Geometry check sheet. Reference: the model listing, model coordinates, mm. Round coordinates to 2 decimals unless told otherwise and drop trailing zeros. Order: outer loops, then holes, each group sorted by start corner. A loop starts at its lowest first (then second) coordinate and runs counter-clockwise, first axis right, second up.
(1) Sectioned sample at C-C (x = -2). Record the boundary of the cut face in (y, z).
(2) Go/stop test with flat-tipped pins: pin 1 (1.5 mm diameter, centred on y = -18.5, z = 42, fed in from -X); pin 2 (6 mm diameter, centred on y = -1, z = 70, fed in from -X); pin 3 (8 mm diameter, centred on x = -19.5, z = 38, fed in from -Y); pin 4 (10 mm diameter, centred on x = 3.5, z = 85, fed in from +Y). Record where each tip stops, or that it passes through.
(3) Material ranges on line 1 along Y through (x, z) = (0, 60); line 2 along Z through (x, y) = (-5, -5); line 3 along Y through (x, z) = (22, 77.5), recorded low to high.
(4) Sectioned sample at A-A (y = 13). Record the boundary of the cut face in (x, z).
(5) Release check for a two-part mould opening along Y. For faces 1 (the face through (22.015, -1.678, 83.496)), 2 (the face through (-22.05, -1.73, 39.43)), 3 (the face through (0.35, -5.206, 54.627)) record: +Y half, -Y half, draft (parallel to the pull), parting line (faces both ways), or undercut.
(6) Sectioned sample at B-B (x = 11). Record the boundary of the cut face in (y, z).
from build123d import *

# Parameters (mm, degrees)
F0_R          = 25
F1_DEPTH      = 140
F1_DEPTH_BACK = 140
F3_DEPTH      = 70
F3_DEPTH_BACK = 70
F4_R          = 4
F5_DEPTH      = 100


with BuildPart() as f1:
    # F0 (on Top) → F1 (new body, two sides)
    with BuildSketch(Plane.XY) as f1_sk:
        Circle(F0_R)
        Polygon((-17.759334, -15.390129), (-17.467051, -11.30056), (-13.377482, -11.592843), (-13.669765, -15.682412), align=None, mode=Mode.SUBTRACT)
        Polygon((-4.986074, -16.984997), (-3.020925, -20.583356), (-6.619284, -22.548505), (-8.584433, -18.950146), align=None, mode=Mode.SUBTRACT)
        Polygon((-12.70393, -19.770184), (-13.575676, -15.763931), (-9.569424, -14.892185), (-8.697678, -18.898437), align=None, mode=Mode.SUBTRACT)
        Polygon((-16.101728, -7.354277), (-17.534361, -11.195835), (-21.375918, -9.763202), (-19.943286, -5.921645), align=None, mode=Mode.SUBTRACT)
        Polygon((-17.52145, -2.519885), (-19.978364, -5.802198), (-23.260677, -3.345284), (-20.803763, -0.062972), align=None, mode=Mode.SUBTRACT)
        Polygon((2.900576, -20.60066), (0.001641, -23.5), (-2.8977, -20.601065), (0.001236, -17.701724), align=None, mode=Mode.SUBTRACT)
        Polygon((8.587079, -18.948947), (6.622432, -22.547581), (3.023799, -20.582934), (4.988446, -16.9843), align=None, mode=Mode.SUBTRACT)
        Polygon((12.70669, -19.76841), (8.700316, -18.897223), (9.571503, -14.890849), (13.577877, -15.762036), align=None, mode=Mode.SUBTRACT)
        Polygon((13.379101, -11.590975), (17.468628, -11.298121), (17.761482, -15.387649), (13.671955, -15.680503), align=None, mode=Mode.SUBTRACT)
        Polygon((21.377281, -9.760218), (17.535924, -11.193387), (16.102755, -7.352029), (19.944112, -5.91886), align=None, mode=Mode.SUBTRACT)
        Polygon((19.979174, -5.799408), (17.521802, -2.517439), (20.803772, -0.060067), (23.261143, -3.342037), align=None, mode=Mode.SUBTRACT)
        Polygon((-23.26091, 3.343661), (-19.978769, 5.800803), (-17.521626, 2.518662), (-20.803767, 0.061519), align=None, mode=Mode.SUBTRACT)
        Polygon((-19.943699, 5.920253), (-21.3766, 9.76171), (-17.535142, 11.194611), (-16.102242, 7.353153), align=None, mode=Mode.SUBTRACT)
        Polygon((-13.67086, 15.681458), (-13.378291, 11.59191), (-17.467839, 11.299341), (-17.760408, 15.388889), align=None, mode=Mode.SUBTRACT)
        Polygon((-9.570464, 14.891517), (-13.576777, 15.762984), (-12.70531, 19.769297), (-8.698997, 18.89783), align=None, mode=Mode.SUBTRACT)
        Polygon((-8.585756, 18.949547), (-6.620858, 22.548043), (-3.022362, 20.583145), (-4.98726, 16.984649), align=None, mode=Mode.SUBTRACT)
        Polygon((19.977959, 5.803593), (23.260443, 3.346908), (20.803759, 0.064424), (17.521274, 2.521108), align=None, mode=Mode.SUBTRACT)
        Polygon((21.375237, 9.764695), (19.942872, 5.923037), (16.101215, 7.355402), (17.533579, 11.197059), align=None, mode=Mode.SUBTRACT)
        Polygon((12.70255, 19.771071), (13.574576, 15.764879), (9.568384, 14.892853), (8.696358, 18.899044), align=None, mode=Mode.SUBTRACT)
        Polygon((-0.00164, 23.49836), (0, 23.5), (2.899138, 20.600862), (0, 17.701724), (-0.001236, 17.70296), (-2.899138, 20.600862), align=None, mode=Mode.SUBTRACT)
        Polygon((6.61771, 22.548967), (8.58311, 18.950745), (4.984888, 16.985345), (3.019488, 20.583567), align=None, mode=Mode.SUBTRACT)
        Polygon((13.376673, 11.593777), (13.66867, 15.683366), (17.758259, 15.391369), (17.466262, 11.30178), align=None, mode=Mode.SUBTRACT)
    extrude(amount=F1_DEPTH)
    extrude(f1_sk.sketch, amount=-F1_DEPTH_BACK)

    # F2 (on Front) → F3 (cut, two sides)
    with BuildSketch(Plane.XZ) as f3_sk:
        Polygon((98.642283, 152.918806), (-61.347591, -7.071068), (-72.7507, -18.474177), (-63.999477, -174.67025), (77.080854, -174.67025), align=None)
        Polygon((-70.218705, 159.989874), (-68.418659, 0), (91.571215, 159.989874), align=None)
    extrude(amount=F3_DEPTH, mode=Mode.SUBTRACT)
    extrude(f3_sk.sketch, amount=-F3_DEPTH_BACK, mode=Mode.SUBTRACT)

    # F4 (on Top) → F5 (cut)
    with BuildSketch(Plane.XY):
        Circle(F4_R)
    extrude(amount=F5_DEPTH, mode=Mode.SUBTRACT)


solid = f1.part
Answer below:
1. outline: (-24.92, 52.28) - (-21.5, 52.28) - (-21.5, 66.42) - (-24.92, 66.42) - close; (-19.7, 52.28) - (-3.46, 52.28) - (-3.46, 66.42) - (-19.7, 66.42) - close; (3.46, 52.28) - (19.7, 52.28) - (19.7, 66.42) - (3.46, 66.42) - close; (21.5, 52.28) - (24.92, 52.28) - (24.92, 66.42) - (21.5, 66.42) - close
2. pin 1: stops at x = -17.61
2. pin 2: stops at x = 0.85
2. pin 3: stops at y = -19.56
2. pin 4: passes through
3. line 1: y = -25 to -23.5, -17.7 to -4, 4 to 17.7, 23.5 to 25
3. line 2: z = 49.28 to 63.42
3. line 3: y = -11.87 to -4.29, -1.66 to 1.66, 4.29 to 11.87
4. outline: (-21.35, 32.92) - (-17.59, 36.69) - (-17.59, 50.83) - (-21.35, 47.06) - close; (-13.48, 40.8) - (13.48, 67.75) - (13.48, 81.9) - (-13.48, 54.94) - close; (17.59, 71.86) - (21.35, 75.63) - (21.35, 89.77) - (17.59, 86.01) - close
5. face 1: undercut
5. face 2: undercut
5. face 3: draft
6. outline: (-22.45, 65.28) - (-19.4, 65.28) - (-19.4, 79.42) - (-22.45, 79.42) - close; (-15.2, 65.28) - (15.2, 65.28) - (15.2, 79.42) - (-15.2, 79.42) - close; (19.4, 65.28) - (22.45, 65.28) - (22.45, 79.42) - (19.4, 79.42) - close
